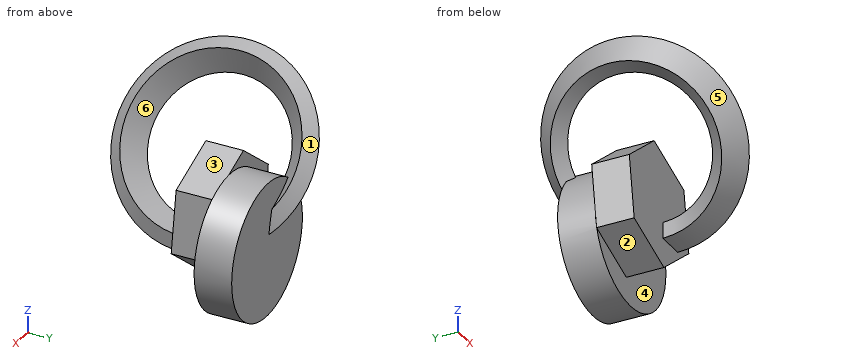
```python
from build123d import *

# Parameters (mm, degrees)
F0_R     = 45.453378
F1_DEPTH = 25.4
F3_DEPTH = 25.4
F4_W     = 19.075925
F4_H     = 10.899786


with BuildPart() as f1:
    # F0 (on Front) → F1 (new body)
    with BuildSketch(Plane.XZ):
        with Locations((-0.326774, -2.101401)):
            Circle(F0_R)
    extrude(amount=F1_DEPTH)

    # F2 (on face) → F3 (join)
    with BuildSketch(Plane.XZ.offset(25.4)):
        Polygon((26.258245, -4.635622), (19.949142, 35.913156), (-18.321682, 50.723701), (-50.283402, 24.985468), (-43.974299, -15.563311), (-5.703475, -30.373856), align=None)
    extrude(amount=F3_DEPTH)

    # F4 (on face) → F5 (revolve)
    with BuildSketch(Plane.XZ.offset(50.8)):
        with Locations((2.4393, -5.449893)):
            Rectangle(F4_W, F4_H)
    revolve(axis=Axis((-34.302542, -50.8, 37.854584), (-0.778858, 0, -0.627201)))


solid = f1.part
```
Read the model definition and answer for the solid it produces. Units are mm, in the model's axes. Face numbers are marked on the shaded views. A direction names the side the tool comes from. Give positions to 0.01 mm unless a question says otherwise; leave off trailing zeros. Write each loop counter-clockwise with the first axis right and the second up, starting at its lowest first coordinate (ties: lowest second). Pieces come first, ordered by that corner, then holes. Notation, with made-up numbers: (32.25, 10.5) -> (74.25, 10.5) arc R21 cw to (74.25, 45.5) -> close; hole circle Ø6 at (54.25, 1). An arc over 180 degrees is marked (long way). Answer in a Markdown table with one row per item.
1) Section A-A on x = -37.5 is taken. Count the separate pieces of the cut face and the enclosed holes in it, plus the area to 3 significant figures.
Results list:
| item | result |
|---|---|
| separate pieces | 3 |
| enclosed holes | 0 |
| area | 3,360 mm^2 |
2) Section C-C on z = -38 is taken. Give the vertices of the cut face in (x, y).
Results list:
| item | result |
|---|---|
| outline | (-28.21, -25.4) -> (27.55, -25.4) -> (27.55, 0) -> (-28.21, 0) -> close |
3) Determine the mould class of the marked faces 4, 5 and 6 for opening direction Y: released by +Y, released by -Y, zero draft, split by the parting line, or undercut.
Results list:
| item | result |
|---|---|
| face 4 | released by -Y |
| face 5 | split by the parting line |
| face 6 | undercut |
4) Each of these flat-tipped pins is pushed along its axis until it touches: pin 1 Ø6 at (x, z) = (-7, 47) entering from +Y; pin 2 Ø5 at (y, z) = (-20.5, -30) entering from +X; pin 3 Ø8 at (y, z) = (-103.5, 4) entering from +X. Where does it stop, or does it pass through?
Results list:
| item | result |
|---|---|
| pin 1 | y = -25.4 |
| pin 2 | x = 37.37 |
| pin 3 | x = -1.47 |
5) A tool of negligible diameter and unlimited length cuts with its end or side. For the marked faces 1, 2 and 3, from which of +Z, -Z, +X, -X, +Y, -Y can it reach the whole face along a straight path? Write none if from no direction.
Results list:
| item | result |
|---|---|
| face 1 | +Z, +X |
| face 2 | -Z, -X, -Y |
| face 3 | +Z, +X, -Y |
6) Straight lines are drawn through the part: line 1 (Y direction, x = -14.5, z = -27.5); line 2 (Y direction, x = -28, z = -4); line 3 (Y direction, x = -28, z = 21). For each, find the intervals that lie inside material, in ascending order. Write a range as [from, to].
Results list:
| item | result |
|---|---|
| line 1 | [-25.4, 0] |
| line 2 | [-50.8, 0] |
| line 3 | [-106.27, -98.22], [-50.8, 4.67] |
